```python
from build123d import *

# Parameters (mm, degrees)
SKETCH2_R           = 6.9
BOSS_EXTRUDE1_DEPTH = 3
SKETCH3_R           = 6.9
SKETCH3_R_2         = 5
BOSS_EXTRUDE2_DEPTH = 53
CHAMFER1_SIZE       = 0.5
CHAMFER2_SIZE       = 1


with BuildPart() as part:
    # Sketch2 → Boss-Extrude1 (new body)
    with BuildSketch(Plane.XY):
        with BuildLine():
            Line((102.765440341, 138.860814374), (120.765440341, 138.860814374))
            ThreePointArc((120.765440341, 138.860814374), (121.472547122, 138.567921155), (121.765440341, 137.860814374))
            Line((121.765440341, 137.860814374), (121.765440341, 118.860814374))
            ThreePointArc((121.765440341, 118.860814374), (120.300974247, 115.325280468), (116.765440341, 113.860814374))
            Line((116.765440341, 113.860814374), (106.765440341, 113.860814374))
            ThreePointArc((106.765440341, 113.860814374), (103.229906435, 115.325280468), (101.765440341, 118.860814374))
            Line((101.765440341, 118.860814374), (101.765440341, 137.860814374))
            ThreePointArc((101.765440341, 137.860814374), (102.058333559, 138.567921155), (102.765440341, 138.860814374))
        make_face()
        with Locations((111.765440341, 128.860814374)):
            Circle(SKETCH2_R, mode=Mode.SUBTRACT)
    extrude(amount=BOSS_EXTRUDE1_DEPTH)

    # Sketch3 → Boss-Extrude2 (add)
    with BuildSketch(Plane.XY):
        with Locations(Location((111.765440341, 128.860814374, 0), (0, 0, 180))):
            Circle(SKETCH3_R)
        with Locations(Location((111.765440341, 128.860814374, 0), (0, 0, 180))):
            Circle(SKETCH3_R_2, mode=Mode.SUBTRACT)
    extrude(amount=BOSS_EXTRUDE2_DEPTH)

    # Chamfer1
    chamfer1_edges = [part.edges().sort_by_distance(p)[0] for p in [
        (121.472547122, 138.567921155, 0),
        (121.765440341, 128.360814374, 0),
        (111.765440341, 138.860814374, 3),
        (120.300974247, 115.325280468, 0),
        (111.765440341, 113.860814374, 0),
        (103.229906435, 115.325280468, 0),
        (101.765440341, 128.360814374, 0),
        (102.058333559, 138.567921155, 0),
        (111.765440341, 138.860814374, 0),
        (102.058333559, 138.567921155, 3),
        (101.765440341, 128.360814374, 3),
        (103.229906435, 115.325280468, 3),
        (118.665440341, 128.860814374, 53),
        (116.765440341, 128.860814374, 0),
        (116.765440341, 128.860814374, 53),
        (111.765440341, 113.860814374, 3),
        (120.300974247, 115.325280468, 3),
        (121.765440341, 128.360814374, 3),
        (121.472547122, 138.567921155, 3),
    ]]
    chamfer(chamfer1_edges, length=CHAMFER1_SIZE)

    # Chamfer2
    chamfer2_edges = [part.edges().sort_by_distance(p)[0] for p in [
        (118.665440341, 128.860814374, 3),
    ]]
    chamfer(chamfer2_edges, length=CHAMFER2_SIZE)


solid = part.part
```
Here's how the part is built. I have some questions about the finished solid (model axes, mm). A direction names the side the tool comes from. Coordinates: 2 decimals unless noted, no trailing zeros. Order: outer loops, then holes, each group sorted by start corner. A loop starts at its lowest first (then second) coordinate and runs counter-clockwise, first axis right, second up. Notation, with made-up numbers: M 5.25,49 L 31.25,49 A23 ccw 31.25,60 Z; hole C 33.5,-17.75 d6. An arc over 180 degrees is marked long. Answer as a JSON object with one key per item and string values. Group by question number.
(1) I need wall thicknesses on probe 1 along Y at (x, z) = (113.5, 33.5); probe 2 along Z at (x, y) = (119.75, 121); probe 3 along Y at (x, z) = (115.25, 21.5). Which ranges of each line are inside material? Lowest first, please.
(2) Suppose I cut it at A-A, the plane z = 18.5. Please give me the cut outline in (x, y), then the cut area to 3 significant figures.
(3) Which directions (+Z, -Z, +X, -X, +Y, -Y) give clear straight access to the entire face, cutting with the end or side of a thin tool? Please do faces 1 (the face through (120.079, 115.619, 2.865)), 2 (the face through (110, 121, 3)).
(4) For pin 1 (12 mm diameter, centred on x = 106, y = 126.5, fed in from -Z); pin 2 (5 mm diameter, centred on x = 114, z = 25, fed in from +Y); pin 3 (1.5 mm diameter, centred on x = 107.5, z = 40.5, fed in from -Y); pin 4 (9 mm diameter, centred on x = 111.77, y = 128.86, fed in from -Z), each with a flat end and sliding along its axis, tell me the tip position at first contact or that it passes through.
Values found:
{
 "1": {"probe 1": "y = 122.18 to 124.17, 133.55 to 135.54", "probe 2": "z = 0 to 3", "probe 3": "y = 122.91 to 125.28, 132.45 to 134.82"},
 "2": {"outline": "C 111.77,128.86 d13.8; hole C 111.77,128.86 d10", "area": "71.0 mm^2"},
 "3": {"face 1": "+Z, +X, -Y", "face 2": "+Z"},
 "4": {"pin 1": "stops at z = 0", "pin 2": "stops at y = 135.76", "pin 3": "stops at y = 122.92", "pin 4": "passes through"}
}
